The listing builds one solid part. Answer for the finished solid, in the listing's coordinates (mm). A direction names the side the tool comes from. Give positions to 0.01 mm unless a question says otherwise; leave off trailing zeros. Write each loop counter-clockwise with the first axis right and the second up, starting at its lowest first coordinate (ties: lowest second). Pieces come first, ordered by that corner, then holes. Notation, with made-up numbers: M 21,54 L 32,54 A20 ccw 32,75 Z; hole C 83.5,46 d10. An arc over 180 degrees is marked long. Answer as a JSON object with one key per item and string values.
```python
from build123d import *

# Parameters (mm, degrees)
ESQUISSE1_W        = 30
ESQUISSE1_H        = 33
BOSS_EXTRU_1_DEPTH = 3
BOSS_EXTRU_2_DEPTH = 18
COQUE1_DEPTH       = 18
ESQUISSE3_W        = 1.5
ESQUISSE3_H        = 3
BOSS_EXTRU_3_DEPTH = 15
CONG_1_R           = 0.5
ESQUISSE4_W        = 27.5
ESQUISSE4_H        = 18
BOSS_EXTRU_4_DEPTH = 10.5
ESQUISSE6_R        = 1.6
BOSS_EXTRU_5_DEPTH = 3
CONG_2_R           = 10
ESQUISSE7_W        = 28.5
ESQUISSE7_H        = 31
BOSS_EXTRU_6_DEPTH = 1.5875


# Read off the part's stored shape, not the designer's step: Coque1
with BuildPart() as part:
    # Esquisse1 → Boss.-Extru.1 (new body)
    with BuildSketch(Plane.XY):
        with Locations((-2.569437515, -9.378787879)):
            Rectangle(ESQUISSE1_W, ESQUISSE1_H)
    extrude(amount=BOSS_EXTRU_1_DEPTH)

    # Esquisse2 → Boss.-Extru.2 (add)
    with BuildSketch(Plane.XY.offset(3)):
        Polygon((-16.319437515, -4.878787879), (11.180562485, -4.878787879), (11.180562485, -18.878787879), (5.680562485, -24.378787879), (-10.819437515, -24.378787879), (-16.319437515, -18.878787879), align=None)
    extrude(amount=BOSS_EXTRU_2_DEPTH)

    # Coque1 outline → Coque1 (cut)
    with BuildSketch(Plane.XY):
        Polygon((-13.319437515, -7.878787879), (-13.319437515, -17.636147192), (-9.576796827, -21.378787879), (4.437921798, -21.378787879), (8.180562485, -17.636147192), (8.180562485, -7.878787879), align=None)
    extrude(amount=COQUE1_DEPTH, mode=Mode.SUBTRACT)

    # Esquisse3 → Boss.-Extru.3 (add)
    with BuildSketch(Plane(origin=(0, 0, 18), x_dir=(-1, 0, 0), z_dir=(0, 0, -1))):
        with Locations((2.569437515, -16.128787879)):
            Rectangle(ESQUISSE3_W, ESQUISSE3_H)
        with Locations((-3.430562485, -13.128787879)):
            Rectangle(ESQUISSE3_W, ESQUISSE3_H)
        with Locations((8.569437515, -13.128787879)):
            Rectangle(ESQUISSE3_W, ESQUISSE3_H)
    extrude(amount=BOSS_EXTRU_3_DEPTH)

    # Congé1
    cong_1_edges = [part.edges().sort_by_distance(p)[0] for p in [
        (-1.819437515, -16.128787879, 3),
        (-2.569437515, -17.628787879, 3),
        (-3.319437515, -16.128787879, 3),
        (-2.569437515, -14.628787879, 3),
        (4.180562485, -13.128787879, 3),
        (3.430562485, -14.628787879, 3),
        (2.680562485, -13.128787879, 3),
        (3.430562485, -11.628787879, 3),
        (-7.819437515, -13.128787879, 3),
        (-8.569437515, -14.628787879, 3),
        (-9.319437515, -13.128787879, 3),
        (-8.569437515, -11.628787879, 3),
    ]]
    fillet(cong_1_edges, radius=CONG_1_R)

    # Esquisse4 → Boss.-Extru.4 (add)
    with BuildSketch(Plane(origin=(0, -4.878787879, 0), x_dir=(1, 0, 0), z_dir=(0, 1, 0))):
        with Locations((-2.569437515, -12)):
            Rectangle(ESQUISSE4_W, ESQUISSE4_H)
    extrude(amount=BOSS_EXTRU_4_DEPTH)

    # Esquisse6 → Boss.-Extru.5 (add)
    # profile 1 of 2: a face of its own
    with BuildSketch(Plane(origin=(0, 0, 0), x_dir=(-1, 0, 0), z_dir=(0, 0, -1))):
        Polygon((17.569437515, -25.878787879), (27.569437515, -10.024052208), (17.569437515, 7.121212121), align=None)
        with Locations((20.569437515, -9.378787879)):
            Circle(ESQUISSE6_R, mode=Mode.SUBTRACT)
    # profile 2 of 2: a face of its own
    with BuildSketch(Plane(origin=(0, 0, 0), x_dir=(-1, 0, 0), z_dir=(0, 0, -1))):
        Polygon((-12.430562485, 7.121212121), (-12.430562485, -25.878787879), (-21.677859795, -10.024052208), align=None)
        with Locations((-15.430562485, -9.378787879)):
            Circle(ESQUISSE6_R, mode=Mode.SUBTRACT)
    extrude(amount=-BOSS_EXTRU_5_DEPTH)

    # Congé2
    cong_2_edges = [part.edges().sort_by_distance(p)[0] for p in [
        (-27.569437515, -10.024052208, 1.5),
        (21.677859795, -10.024052208, 1.5),
    ]]
    fillet(cong_2_edges, radius=CONG_2_R)

    # Esquisse7 → Boss.-Extru.6 (add)
    with BuildSketch(Plane(origin=(0, 0, 0), x_dir=(-1, 0, 0), z_dir=(0, 0, -1))):
        with Locations((2.569437515, -9.378787879)):
            Rectangle(ESQUISSE7_W, ESQUISSE7_H)
        Polygon((-4.437921798, -21.378787879), (-8.180562485, -17.636147192), (-8.180562485, -7.878787879), (13.319437515, -7.878787879), (13.319437515, -17.636147192), (9.576796827, -21.378787879), align=None, mode=Mode.SUBTRACT)
    extrude(amount=BOSS_EXTRU_6_DEPTH)


solid = part.part
```
1. A cutting plane is placed at C-C, the plane y = 5. Give the vertices of the cut face in (x, z), plus the area to 3 significant figures.
Verdict:
{"outline": "M -18.81,0 L -16.82,0 L -16.82,-1.59 L 11.68,-1.59 L 11.68,0 L 13.57,0 L 13.57,3 L 11.18,3 L 11.18,21 L -16.32,21 L -16.32,3 L -18.81,3 Z", "area": "637 mm2"}
2. Consider line 1 along X through (y, z) = (-17, 14.75); line 2 along Y through (x, z) = (3.5, 7.5); line 3 along X through (y, z) = (-13.5, 5.25). Determine where each line is inside the solid, lowest interval first.
Verdict:
{"line 1": "x = -16.32 to -13.32, -3.32 to -1.82, 8.18 to 11.18", "line 2": "y = -24.38 to -21.38, -14.63 to -11.63, -7.88 to 5.62", "line 3": "x = -16.32 to -13.32, -9.32 to -7.82, 2.68 to 4.18, 8.18 to 11.18"}
3. A cutting plane is placed at B-B, the plane x = -7. Give the vertices of the cut face in (y, z), plus the area to 3 significant figures.
Verdict:
{"outline": "M -25.88,0 L -24.88,0 L -24.88,-1.59 L -21.38,-1.59 L -21.38,18 L -7.88,18 L -7.88,-1.59 L 6.12,-1.59 L 6.12,0 L 7.12,0 L 7.12,3 L 5.62,3 L 5.62,21 L -24.38,21 L -24.38,3 L -25.88,3 Z", "area": "424 mm2"}
4. Flat-ended cylindrical pins translate along their axes: pin 1 (4 mm diameter, centred on x = -7.5, z = 7.5, fed in from +Y); pin 2 (6 mm diameter, centred on y = 1.5, z = 15.5, fed in from +X); pin 3 (3 mm diameter, centred on y = 3, z = 1.5, fed in from -X). Find the tip coordinate at first contact, or state that the pin passes through.
Verdict:
{"pin 1": "stops at y = 5.62", "pin 2": "stops at x = 11.18", "pin 3": "stops at x = -20.85"}
5. The mould has two halves that part along Y. Classify faces 5 (the flat face through (-16.819, -10, -1)), 6 (the flat face through (-3.319, -16, 11)), 7 (the flat face through (-2, -24.879, -1)): released by +Y, released by -Y, zero draft, split by the parting line, or undercut.
Verdict:
{"face 5": "zero draft", "face 6": "undercut", "face 7": "released by -Y"}
6. For faces 1 (the flat face through (-3, 5.621, 12)), 2 (the flat face through (-9.319, -13, 11)), 3 (the flat face through (-2, 6.121, -1)), 4 (the flat face through (-2, -24.379, 12)), determine the directions among +Z, -Z, +X, -X, +Y, -Y from which every point of the face is accessible in a straight line to the end or side of a thin tool.
Verdict:
{"face 1": "+Z, +X, -X, +Y", "face 2": "-Z", "face 3": "-Z, +X, -X, +Y", "face 4": "+Z, +X, -X, -Y"}
7. A cutting plane is placed at A-A, the plane z = 12.25. Give the vertices of the cut face in (x, y), plus the area to 3 significant figures.
Verdict:
{"outline": "M -16.32,-18.88 L -10.82,-24.38 L 5.68,-24.38 L 11.18,-18.88 L 11.18,5.62 L -16.32,5.62 Z; M -9.32,-14.63 L -7.82,-14.63 L -7.82,-11.63 L -9.32,-11.63 Z; M -3.32,-17.63 L -1.82,-17.63 L -1.82,-14.63 L -3.32,-14.63 Z; M 2.68,-14.63 L 4.18,-14.63 L 4.18,-11.63 L 2.68,-11.63 Z; hole M -13.32,-17.64 L -9.58,-21.38 L 4.44,-21.38 L 8.18,-17.64 L 8.18,-7.88 L -13.32,-7.88 Z", "area": "532 mm2"}
8. A cutting plane is placed at D-D, the plane z = 19.5. Give the vertices of the cut face in (x, y), plus the area to 3 significant figures.
Verdict:
{"outline": "M -16.32,-18.88 L -10.82,-24.38 L 5.68,-24.38 L 11.18,-18.88 L 11.18,5.62 L -16.32,5.62 Z", "area": "795 mm2"}
